```python
from build123d import *

# Parameters (mm, degrees)
F0_W       = 5
F0_H       = 3
F0_W_2     = 20
F1_DEPTH   = 3
F2_DEPTH   = 3
F3_SIZE2   = 4.99999
F3_SIZE    = 2.99999
F3_2_SIZE2 = 4.99999
F3_2_SIZE  = 2.99999


# Not quite as in the source:
# - a fillet or chamfer is up to 0.001 mm smaller than in the source, because OpenCascade refuses the exact size


with BuildPart() as f1:
    # F0 (on Top) → F1 (new body)
    with BuildSketch(Plane.XY):
        with BuildLine():
            Line((16.5, 10), (-16.5, 10))
            ThreePointArc((-16.5, 10), (-20.0355339059, 8.5355339059), (-21.5, 5))
            ThreePointArc((-21.5, 5), (-20.0355339059, 1.4644660941), (-16.5, 0))
            Line((-16.5, 0), (16.5, 0))
            ThreePointArc((16.5, 0), (20.0355339059, 1.4644660941), (21.5, 5))
            ThreePointArc((21.5, 5), (20.0355339059, 8.5355339059), (16.5, 10))
        make_face()
        with Locations((-15.5, 5)):
            Rectangle(F0_W, F0_H, mode=Mode.SUBTRACT)
        with Locations((0, 5)):
            Rectangle(F0_W_2, F0_H, mode=Mode.SUBTRACT)
        with Locations((15.5, 5)):
            Rectangle(F0_W, F0_H, mode=Mode.SUBTRACT)
        with Locations((0, 5)):
            Rectangle(F0_W_2, F0_H)
    extrude(amount=F1_DEPTH)

    # F0 (on Top) → F2 (join)
    with BuildSketch(Plane.XY):
        with Locations((0, 5)):
            Rectangle(F0_W_2, F0_H)
    extrude(amount=-F2_DEPTH)

    # F3 (size 3 and 5 in the source; OpenCascade refuses exactly that, so slightly less here)
    f3_edges = [f1.edges().sort_by_distance(p)[0] for p in [
        (-10, 5, -3),
    ]]
    f3_side = f1.faces().sort_by_distance((-10, 5, -1.5))[0]
    chamfer(f3_edges, length=F3_SIZE, length2=F3_SIZE2, reference=f3_side)

    # F3#2 (size 3 and 5 in the source; OpenCascade refuses exactly that, so slightly less here)
    f3_2_edges = [f1.edges().sort_by_distance(p)[0] for p in [
        (10, 5, -3),
    ]]
    f3_2_side = f1.faces().sort_by_distance((10, 5, -1.5))[0]
    chamfer(f3_2_edges, length=F3_2_SIZE, length2=F3_2_SIZE2, reference=f3_2_side)


solid = f1.part
```
CAD build for the part. Positions are in the model's coordinates, mm. A direction names the side the tool comes from. Round coordinates to 2 decimals unless told otherwise and drop trailing zeros. Order: outer loops, then holes, each group sorted by start corner. A loop starts at its lowest first (then second) coordinate and runs counter-clockwise, first axis right, second up.
Item 1: Mould opens along X. For faces 1 (the face through (15, 6.5, 1)), 2 (the face through (7.5, 5, -1.5)), 3 (the face through (18, 5, 1)), 4 (the face through (0, 3, 0)) say: pulls with the +X half, pulls with the -X half, needs draft (parallel to the pull), parting line crosses it, or undercut.
Item 2: Saw through at B-B on x = -7. Write the cut outline in (y, z), then the cut area to 3 significant figures.
Item 3: Saw through at C-C on y = 8. Write the cut outline in (x, z).
Item 4: Saw through at A-A on z = 1.8. Write the cut outline in (x, y), then the cut area to 3 significant figures.
Item 5: Saw through at D-D on x = 2.5. Write the cut outline in (y, z).
Item 6: Tool access for faces 5 (the face through (0, 6.5, -1)), 6 (the face through (13, 5, 1)), 7 (the face through (0, 3.5, -1)): list every direction of +Z, -Z, +X, -X, +Y, -Y with a clear straight run to the whole face (end or side of a thin tool).
Item 7: Pin check, flat tips, straight feed: pin 1 (1.5 mm diameter, centred on x = 3.5, y = 2.5, fed in from -Z); pin 2 (0.9 mm diameter, centred on x = -4.5, z = -1, fed in from -Y); pin 3 (1 mm diameter, centred on y = 7, z = 2, fed in from +X). Stop position of each tip, or through.
Item 8: Probe line 1 along X through (y, z) = (4.5, 2.4); line 2 along X through (y, z) = (6.25, 1.25); line 3 along Z through (x, y) = (-11.5, 2.5). List the from-to ranges inside material, lowest first.
Reported:
1. face 1: undercut
1. face 2: pulls with the +X half
1. face 3: undercut
1. face 4: needs draft
2. outline: (0, 0) - (3.5, 0) - (3.5, -1.8) - (6.5, -1.8) - (6.5, 0) - (10, 0) - (10, 3) - (0, 3) - close
2. area: 35.4 mm2
3. outline: (-20.5, 0) - (20.5, 0) - (20.5, 3) - (-20.5, 3) - close
4. outline: (-16.5, 0) - (16.5, 0) arc R5 ccw to (16.5, 10) - (-16.5, 10) arc R5 ccw to start; hole (-18, 3.5) - (-13, 3.5) - (-13, 6.5) - (-18, 6.5) - close; hole (13, 3.5) - (18, 3.5) - (18, 6.5) - (13, 6.5) - close
4. area: 379 mm2
5. outline: (0, 0) - (3.5, 0) - (3.5, -3) - (6.5, -3) - (6.5, 0) - (10, 0) - (10, 3) - (0, 3) - close
6. face 5: -Z, +X, -X, +Y
6. face 6: +Z, -Z
6. face 7: -Z, +X, -X, -Y
7. pin 1: stops at z = 0
7. pin 2: stops at y = 3.5
7. pin 3: stops at x = 21.27
8. line 1: x = -21.47 to -18, -13 to 13, 18 to 21.47
8. line 2: x = -21.34 to -18, -13 to 13, 18 to 21.34
8. line 3: z = 0 to 3
